Geometry: final body of the model. Coordinates: model frame, mm. Face numbers are marked on the shaded views. A direction names the side the tool comes from. Give positions to 0.01 mm unless a question says otherwise; leave off trailing zeros. Order: outer loops, then holes, each group sorted by start corner. A loop starts at its lowest first (then second) coordinate and runs counter-clockwise, first axis right, second up. Notation, with made-up numbers: (35, 51) -> (40, 51) arc R23 ccw to (40, 61) -> close; hole circle Ø3 at (-39, 47.25). An arc over 180 degrees is marked (long way). Answer in a Markdown table with one row per item. Add a question column.
Q1. Set-up query: the marked faces 4, 5 and 6. Return all of +Z, -Z, +X, -X, +Y, -Y with unobstructed straight access to the full face (end or side cutting, diameter ignored); none if empty.
Q2. Cut plane A-A on y = 0. Return the cut outline in (x, z), and give its area (3 significant figures).
Q3. Cut plane B-B on x = 3. Return the cut outline in (y, z).
Q4. Pull-direction query (X, two-part tool) for the marked faces 1, 2 and 3; classes: +X half, -X half, draft (parallel to the pull), parting line (faces both ways), or undercut.
Q5. Cut plane C-C on z = 12.5. Return the cut outline in (x, y).
Q6. Contact query for flat-ended pins moving along their axis: P1, Ø1.5, axis at x = 3.5, z = -14, coming from the -Y side; P2, Ø2, axis at x = -1, z = -14.5, coming from the -Y side; P3, Ø1.5, axis at x = 2, y = 1.5, coming from the -Z side; P4, Ø2, axis at y = -12, z = -12.5, coming from the -X side. Output: stop coordinate, or through.
Q7. Cut plane D-D on x = -5.5. Return the cut outline in (y, z).
Q8. Line query: line 1 along Y through (x, z) = (0, 23); line 2 along Y through (x, z) = (0, -18.5); line 3 along Z through (x, y) = (-12.5, 5). Output: solid intervals per line, ascending. Write a range as from..to.
from build123d import *

# Parameters (mm, degrees)
F0_R     = 9.349188324
F0_R_2   = 6.6042884463
F0_R_3   = 4.4026997979
F1_DEPTH = 6.35
F0_R_4   = 2.4090089184
F2_DEPTH = 31.75
F3_DEPTH = 25.4


# Not quite as in the source:
# - a length typed as a fraction of an inch, garbled in the dataset ("3 / 203.2 mm" for 3/8 in), is restored


with BuildPart() as f1:
    # F0 (on Top) → F1 (new body)
    with BuildSketch(Plane.XY):
        Polygon((15.0401592255, -8.6834399775), (15.0401592255, 8.6834399775), (0, 17.366879955), (-15.0401592255, 8.6834399775), (-15.0401592255, -8.6834399775), (0, -17.366879955), align=None)
        Circle(F0_R, mode=Mode.SUBTRACT)
        Circle(F0_R)
        Circle(F0_R_2, mode=Mode.SUBTRACT)
        Circle(F0_R_2)
        Circle(F0_R_3, mode=Mode.SUBTRACT)
    extrude(amount=F1_DEPTH)

    # F0 (on Top) → F2 (join)
    with BuildSketch(Plane.XY):
        Circle(F0_R_3)
        Circle(F0_R_4, mode=Mode.SUBTRACT)
    extrude(amount=F2_DEPTH)

    # F0 (on Top) → F3 (join)
    with BuildSketch(Plane.XY):
        Circle(F0_R)
        Circle(F0_R_2, mode=Mode.SUBTRACT)
    extrude(amount=-F3_DEPTH)


solid = f1.part
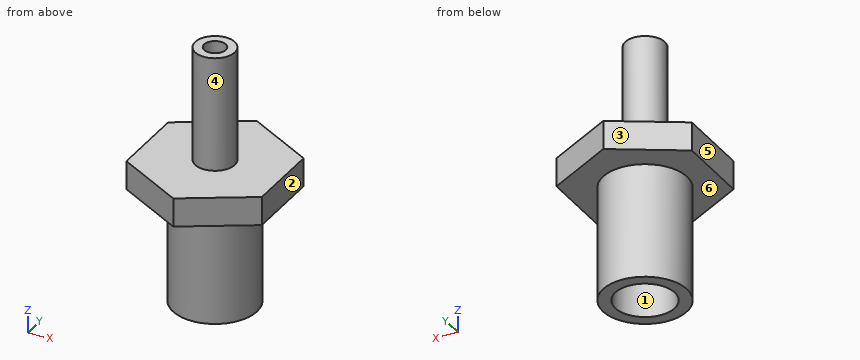
Completed:
| question | item | result |
|---|---|---|
| 1 | face 4 | +Z |
| 1 | face 5 | +Z, -Z, -X, +Y, -Y |
| 1 | face 6 | -Z |
| 2 | outline | (-15.04, 0) -> (-9.35, 0) -> (-9.35, -25.4) -> (-6.6, -25.4) -> (-6.6, 0) -> (-2.41, 0) -> (-2.41, 31.75) -> (-4.4, 31.75) -> (-4.4, 6.35) -> (-15.04, 6.35) -> close; (2.41, 0) -> (6.6, 0) -> (6.6, -25.4) -> (9.35, -25.4) -> (9.35, 0) -> (15.04, 0) -> (15.04, 6.35) -> (4.4, 6.35) -> (4.4, 31.75) -> (2.41, 31.75) -> close |
| 2 | area | 401 mm² |
| 3 | outline | (-15.63, 0) -> (-8.85, 0) -> (-8.85, -25.4) -> (-5.88, -25.4) -> (-5.88, 0) -> (5.88, 0) -> (5.88, -25.4) -> (8.85, -25.4) -> (8.85, 0) -> (15.63, 0) -> (15.63, 6.35) -> (3.22, 6.35) -> (3.22, 31.75) -> (-3.22, 31.75) -> (-3.22, 6.35) -> (-15.63, 6.35) -> close |
| 4 | face 1 | undercut |
| 4 | face 2 | +X half |
| 4 | face 3 | -X half |
| 5 | outline | circle Ø8.81 at (0, 0); hole circle Ø4.82 at (0, 0) |
| 6 | P1 | stops at y = -8.94 |
| 6 | P2 | stops at y = -9.35 |
| 6 | P3 | stops at z = 0 |
| 6 | P4 | passes through |
| 7 | outline | (-14.19, 0) -> (-7.56, 0) -> (-7.56, -25.4) -> (-3.66, -25.4) -> (-3.66, 0) -> (3.66, 0) -> (3.66, -25.4) -> (7.56, -25.4) -> (7.56, 0) -> (14.19, 0) -> (14.19, 6.35) -> (-14.19, 6.35) -> close |
| 8 | line 1 | y = -4.4..-2.41, 2.41..4.4 |
| 8 | line 2 | y = -9.35..-6.6, 6.6..9.35 |
| 8 | line 3 | z = 0..6.35 |
